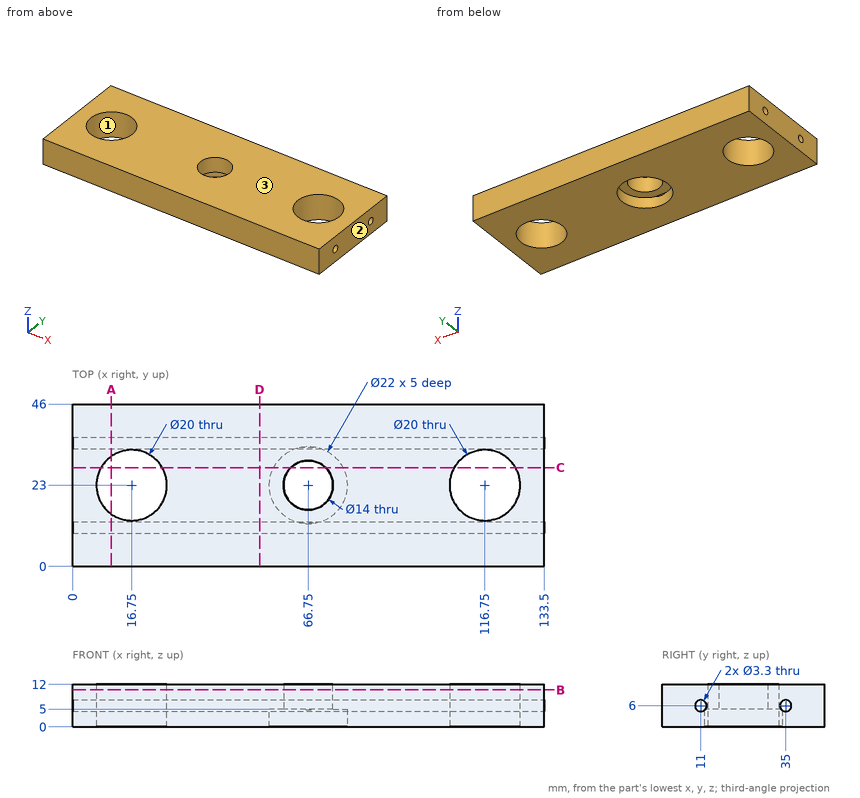
Geometry: see drawing. Coordinates: mm, zero at the bounding-box minimum. Round coordinates to 2 decimals unless told otherwise and drop trailing zeros. Write each loop counter-clockwise with the first axis right and the second up, starting at its lowest first coordinate (ties: lowest second). Pieces come first, ordered by that corner, then holes.
1) Contact query for flat-ended pins moving along their axis: P1, Ø6, axis at x = 64.5, z = 6.5, coming from the -Y side; P2, Ø3, axis at y = 35, z = 6, coming from the -X side. Output: stop coordinate, or through.
2) Cut plane D-D (x = 53). Return the cut outline in (y, z).
3) Ray query, L1, parallel to Y at x = 66.75, z = 2.2; L2, parallel to Y at x = 16.75, z = 8.5; L3, parallel to X at y = 31, z = 5.5. Return the intervals inside material, ascending.
4) Cut plane A-A (x = 11). Return the cut outline in (y, z), then the cut area to 3 significant figures.
5) Cut plane C-C (y = 28). Return the cut outline in (x, z), then the cut area to 3 significant figures.
6) Cut plane B-B (z = 10.5). Return the cut outline in (x, y).
7) Draft query along X for the marked faces 1, 2 and 3. Return one class per face: pulls with the +X half, pulls with the -X half, needs draft (parallel to the pull), parting line crosses it, or undercut.
Geometry says:
1. P1: stops at y = 0
1. P2: passes through
2. outline: (0, 0) - (46, 0) - (46, 12) - (0, 12) - close; hole circle Ø3.3 at (11, 6); hole circle Ø3.3 at (35, 6)
3. L1: y = 0 to 12, 34 to 46
3. L2: y = 0 to 13, 33 to 46
3. L3: x = 0 to 10.75, 22.75 to 110.75, 122.75 to 133.5
4. outline: (0, 0) - (14.82, 0) - (14.82, 12) - (0, 12) - close; (31.18, 0) - (46, 0) - (46, 12) - (31.18, 12) - close; hole circle Ø3.3 at (11, 6); hole circle Ø3.3 at (35, 6)
4. area: 339 mm2
5. outline: (0, 0) - (8.09, 0) - (8.09, 12) - (0, 12) - close; (25.41, 0) - (56.95, 0) - (56.95, 5) - (61.85, 5) - (61.85, 12) - (25.41, 12) - close; (71.65, 5) - (76.55, 5) - (76.55, 0) - (108.09, 0) - (108.09, 12) - (71.65, 12) - close; (125.41, 0) - (133.5, 0) - (133.5, 12) - (125.41, 12) - close
5. area: 1,020 mm2
6. outline: (0, 0) - (133.5, 0) - (133.5, 46) - (0, 46) - close; hole circle Ø20 at (16.75, 23); hole circle Ø14 at (66.75, 23); hole circle Ø20 at (116.75, 23)
7. face 1: undercut
7. face 2: pulls with the +X half
7. face 3: needs draft
